Could you check a few things on this model? Use its own coordinates, in mm. A direction names the side the tool comes from. Coordinates: 2 decimals unless noted, no trailing zeros. Order: outer loops, then holes, each group sorted by start corner. A loop starts at its lowest first (then second) coordinate and runs counter-clockwise, first axis right, second up. Notation, with made-up numbers: (53.25, 62) -> (87.25, 62) arc R20 cw to (87.25, 86) -> close; hole circle Ø10 at (-29.5, 63.25). An arc over 180 degrees is marked (long way). Use a Markdown table: item, result. Add a question column.
1) Will these pins go through, and if not, where does the flat tip stop? pin 1 Ø1 at (x, z) = (1086.5, 212.5) entering from -Y; pin 2 Ø10 at (x, y) = (818, 769.5) entering from +Z; pin 3 Ø10 at (x, y) = (903.5, 157) entering from -Z; pin 4 Ø3 at (y, z) = (604, 85) entering from -X.
2) If I drill on L1, parallel to X at y = 150, z = 58.5; L2, parallel to Y at x = 3.5, z = 29; L3, parallel to X at y = 205.5, z = 50, over which ranges is the centre line in solid material (lowest first)? Write a range as [from, to].
3) If we section it at D-D (y = -7.5): Write out the boundary of the cut face in (x, z).
4) If we section it at B-B (z = 433): Write out the boundary of the cut face in (x, y), plus the area to 3 significant figures.
5) If we section it at C-C (x = 110.5): Write out the boundary of the cut face in (y, z), plus the area to 3 significant figures.
6) Which directions (+Z, -Z, +X, -X, +Y, -Y) give clear straight access to the entire face, cutting with the end or side of a thin tool? Please do faces 1 (the flat face through (-5, 607.5, 126)), 2 (the flat face through (1130, 759, 259)), 3 (the flat face through (1184, 439, 250)), 4 (the flat face through (305, 426.5, 139)).
7) If we section it at A-A (x = 883.5): Write out the boundary of the cut face in (y, z), plus the area to 3 significant figures.
8) Thinking about a two-plate mould opening in X: for faces 5 (the flat face through (794, 603, 139)), 6 (the flat face through (-25, 9, 251)), 7 (the flat face through (599, -25, 79)), which applies, +X half, -X half, draft (parallel to the pull), parting line (faces both ways), or undercut?
```python
from build123d import *

# Parameters (mm, degrees)
F0_W     = 179
F0_H     = 12
F0_W_2   = 138
F0_H_2   = 40
F0_W_3   = 40
F0_H_3   = 120
F0_W_4   = 92
F0_W_5   = 12
F0_H_4   = 90
F0_H_5   = 180
F0_W_6   = 87
F0_H_6   = 92
F0_W_7   = 26
F0_H_7   = 142
F0_H_8   = 136
F0_W_8   = 228
F0_H_9   = 18
F0_H_10  = 20
F0_W_9   = 20
F1_DEPTH = 5
F2_DEPTH = 277
F3_W     = 40
F3_H     = 120
F3_H_2   = 180
F4_DEPTH = 27
F6_DEPTH = 70
F7_DEPTH = 1265
F8_DEPTH = 70


with BuildPart() as f1:
    # F0 (on Top) → F1 (new body)
    with BuildSketch(Plane.XY):
        with Locations((1040.5, 269)):
            Rectangle(F0_W, F0_H)
        Polygon((794, 408), (794, 420), (669, 420), (669, 515), (652, 515), (652, 503), (657, 503), (657, 408), align=None)
        with Locations((392, -5)):
            Rectangle(F0_W_2, F0_H_2)
        Polygon((1130, 350), (1130, 530), (1130, 780), (806, 780), (806, 691), (832, 691), (832, 549), (806, 549), (806, 385), (806, 293), (806, 275), (839, 275), (859, 275), (951, 275), (1130, 275), align=None)
        with Locations((-5, 547.5)):
            Rectangle(F0_W_3, F0_H_3)
        with Locations((-5, 247.5)):
            Rectangle(F0_W_3, F0_H_3)
        Polygon((15, 487.5), (-25, 487.5), (-25, 307.5), (15, 307.5), (15, 382.1609020233), (15, 391.5), (15, 403.5), align=None)
        Polygon((15, 187.5), (-25, 187.5), (-25, -25), (323, -25), (323, 15), (15, 15), align=None)
        Polygon((1130, 15), (1130, 263), (951, 263), (859, 263), (839, 263), (839, 243), (839, 151), (839, 15), align=None)
        with Locations((905, 269)):
            Rectangle(F0_W_4, F0_H)
        Polygon((364.8940163038, 391.5), (243, 391.5), (243, 382.5), (364.8667633533, 382.5), align=None)
        Polygon((473, 780), (461, 780), (461, 498.5), (473, 498.5), (473, 503), (473, 515), align=None)
        with Locations((467, 453.5)):
            Rectangle(F0_W_5, F0_H_4)
        Polygon((243, 426.5), (243, 403.5), (364.9303535711, 403.5), (365, 426.5), align=None)
        Polygon((473, 503), (473, 498.5), (473, 408.5), (473, 386.5), (473, 296.5), (473, 275), (653, 275), (670, 275), (794, 275), (794, 293), (794, 385), (794, 408), (657, 408), (657, 503), (652, 503), (560, 503), align=None)
        with Locations((1150, 440)):
            Rectangle(F0_W_3, F0_H_5)
        Polygon((665, 263), (665, 15), (827, 15), (827, 151), (827, 243), (827, 263), (806, 263), (794, 263), align=None)
        with Locations((516.5, 509)):
            Rectangle(F0_W_6, F0_H)
        with Locations((467, 341.5)):
            Rectangle(F0_W_5, F0_H_4)
        Polygon((15, 382.1609020233), (15, 307.5), (15, 187.5), (15, 15), (323, 15), (461, 15), (461, 198.5), (435, 198.5), (435, 262.5), (461, 262.5), (461, 296.5), (461, 386.5), (461, 391.5), (365, 391.5), (364.8940163038, 391.5), (364.8667633533, 382.5), (243, 382.5), (243, 391.5), (15, 391.5), align=None)
        Polygon((1170, 530), (1170, 820), (-25, 820), (-25, 607.5), (15, 607.5), (15, 780), (461, 780), (473, 780), (794, 780), (806, 780), (1130, 780), (1130, 530), align=None)
        with Locations((833, 197)):
            Rectangle(F0_W_5, F0_H_6)
        Polygon((461, 198.5), (461, 15), (473, 15), (473, 275), (473, 296.5), (461, 296.5), (461, 262.5), (435, 262.5), (435, 198.5), align=None)
        Polygon((794, 420), (794, 780), (473, 780), (473, 515), (560, 515), (652, 515), (669, 515), (669, 420), align=None)
        with Locations((819, 620)):
            Rectangle(F0_W_7, F0_H_7)
        with Locations((606, 509)):
            Rectangle(F0_W_4, F0_H)
        with Locations((833, 83)):
            Rectangle(F0_W_5, F0_H_8)
        Polygon((653, 275), (653, 15), (665, 15), (665, 263), (794, 263), (794, 275), (670, 275), align=None)
        Polygon((1170, -25), (1170, 350), (1130, 350), (1130, 275), (1130, 263), (1130, 15), (839, 15), (827, 15), (665, 15), (653, 15), (473, 15), (461, 15), (461, -25), align=None)
        with Locations((800, 339)):
            Rectangle(F0_W_5, F0_H_6)
        with Locations((129, 397.5)):
            Rectangle(F0_W_8, F0_H)
        with Locations((800, 284)):
            Rectangle(F0_W_5, F0_H_9)
        Polygon((806, 691), (806, 780), (794, 780), (794, 420), (794, 408), (794, 385), (806, 385), (806, 549), align=None)
        with Locations((833, 253)):
            Rectangle(F0_W_5, F0_H_10)
        Polygon((839, 263), (839, 275), (806, 275), (806, 263), (827, 263), align=None)
        with Locations((849, 269)):
            Rectangle(F0_W_9, F0_H)
        Polygon((365, 403.5), (364.9303535711, 403.5), (364.8940163038, 391.5), (365, 391.5), (461, 391.5), (461, 386.5), (473, 386.5), (473, 408.5), (461, 408.5), (461, 403.5), align=None)
        Polygon((364.9303535711, 403.5), (243, 403.5), (243, 391.5), (364.8940163038, 391.5), align=None)
        with Locations((800, 269)):
            Rectangle(F0_W_5, F0_H)
        Polygon((15, 780), (15, 607.5), (15, 487.5), (15, 403.5), (243, 403.5), (243, 426.5), (365, 426.5), (364.9303535711, 403.5), (365, 403.5), (461, 403.5), (461, 408.5), (461, 498.5), (461, 780), align=None)
    extrude(amount=F1_DEPTH)

    # F0 (on Top) → F2 (join)
    with BuildSketch(Plane.XY):
        Polygon((15, 187.5), (-25, 187.5), (-25, -25), (323, -25), (323, 15), (15, 15), align=None)
        with Locations((392, -5)):
            Rectangle(F0_W_2, F0_H_2)
        Polygon((1170, -25), (1170, 350), (1130, 350), (1130, 275), (1130, 263), (1130, 15), (839, 15), (827, 15), (665, 15), (653, 15), (473, 15), (461, 15), (461, -25), align=None)
        with Locations((833, 83)):
            Rectangle(F0_W_5, F0_H_8)
        Polygon((653, 275), (653, 15), (665, 15), (665, 263), (794, 263), (794, 275), (670, 275), align=None)
        Polygon((461, 198.5), (461, 15), (473, 15), (473, 275), (473, 296.5), (461, 296.5), (461, 262.5), (435, 262.5), (435, 198.5), align=None)
        Polygon((15, 487.5), (-25, 487.5), (-25, 307.5), (15, 307.5), (15, 382.1609020233), (15, 391.5), (15, 403.5), align=None)
        with Locations((129, 397.5)):
            Rectangle(F0_W_8, F0_H)
        Polygon((243, 426.5), (243, 403.5), (364.9303535711, 403.5), (365, 426.5), align=None)
        Polygon((364.9303535711, 403.5), (243, 403.5), (243, 391.5), (364.8940163038, 391.5), align=None)
        Polygon((364.8940163038, 391.5), (243, 391.5), (243, 382.5), (364.8667633533, 382.5), align=None)
        Polygon((365, 403.5), (364.9303535711, 403.5), (364.8940163038, 391.5), (365, 391.5), (461, 391.5), (461, 386.5), (473, 386.5), (473, 408.5), (461, 408.5), (461, 403.5), align=None)
        Polygon((473, 780), (461, 780), (461, 498.5), (473, 498.5), (473, 503), (473, 515), align=None)
        with Locations((516.5, 509)):
            Rectangle(F0_W_6, F0_H)
        Polygon((794, 408), (794, 420), (669, 420), (669, 515), (652, 515), (652, 503), (657, 503), (657, 408), align=None)
        Polygon((806, 691), (806, 780), (794, 780), (794, 420), (794, 408), (794, 385), (806, 385), (806, 549), align=None)
        with Locations((833, 253)):
            Rectangle(F0_W_5, F0_H_10)
        with Locations((849, 269)):
            Rectangle(F0_W_9, F0_H)
        Polygon((839, 263), (839, 275), (806, 275), (806, 263), (827, 263), align=None)
        with Locations((800, 269)):
            Rectangle(F0_W_5, F0_H)
        with Locations((800, 284)):
            Rectangle(F0_W_5, F0_H_9)
        with Locations((1040.5, 269)):
            Rectangle(F0_W, F0_H)
        Polygon((1170, 530), (1170, 820), (-25, 820), (-25, 607.5), (15, 607.5), (15, 780), (461, 780), (473, 780), (794, 780), (806, 780), (1130, 780), (1130, 530), align=None)
        with Locations((819, 620)):
            Rectangle(F0_W_7, F0_H_7)
    extrude(amount=F2_DEPTH)

    # F3 (on face) → F4 (join)
    with BuildSketch(Plane.XY.offset(277)):
        with Locations((-5, 547.5)):
            Rectangle(F3_W, F3_H)
        with Locations((-5, 397.5)):
            Rectangle(F3_W, F3_H_2)
        with Locations((-5, 247.5)):
            Rectangle(F3_W, F3_H)
        with Locations((1150, 440)):
            Rectangle(F3_W, F3_H_2)
    extrude(amount=-F4_DEPTH)

    # F5 (on face) → F6 (join)
    with BuildSketch(Plane(origin=(-25, 0, 0), x_dir=(0, -1, 0), z_dir=(-1, 0, 0))):
        Polygon((-365.5990801838, 496), (-397.5, 496), (-125.3602941176, 277), (-93.4593743014, 277), align=None)
        Polygon((-93.4593743014, 277), (-125.3602941176, 277), (25, 156), (25, 181.6717461243), align=None)
        Polygon((25, 181.6717461243), (25, 156), (146.7794117647, 58), (159.3182351687, 73.5813320241), align=None)
        Polygon((-429.4009198162, 496), (-397.5, 496), (-365.5990801838, 496), (-397.5, 521.6717461243), align=None)
        Polygon((-669.6397058824, 277), (-397.5, 496), (-429.4009198162, 496), (-701.5406256986, 277), align=None)
        Polygon((-941.7794117647, 58), (-820, 156), (-820, 181.6717461243), (-954.3182351687, 73.5813320241), align=None)
        Polygon((-820, 156), (-669.6397058824, 277), (-701.5406256986, 277), (-820, 181.6717461243), align=None)
    extrude(amount=F6_DEPTH)

    # F7 (add, through all): a face of the model
    f7_faces = [f1.faces().sort_by_distance(p)[0] for p in [
        (-95, 117.7974560425, 286.3979384905),
    ]]
    extrude(f7_faces, amount=-F7_DEPTH)

    # F8 (add): a face of the model
    f8_faces = [f1.faces().sort_by_distance(p)[0] for p in [
        (1170, 807.7023270544, 229.3358730621),
    ]]
    extrude(f8_faces, amount=F8_DEPTH)


solid = f1.part
```
Answer sheet:
| question | item | result |
|---|---|---|
| 1 | pin 1 | y = -25 |
| 1 | pin 2 | z = 226.33 |
| 1 | pin 3 | z = 0 |
| 1 | pin 4 | x = 461 |
| 2 | L1 | [-25, 15], [461, 473], [653, 665], [827, 839], [1130, 1240] |
| 2 | L2 | [-25, 187.5], [307.5, 487.5], [607.5, 820] |
| 2 | L3 | [435, 473], [653, 665], [1130, 1240] |
| 3 | outline | (-95, 170.08) -> (-25, 170.08) -> (-25, 0) -> (1240, 0) -> (1240, 277) -> (-25, 277) -> (-25, 195.75) -> (-95, 195.75) -> close |
| 4 | outline | (-95, 287.31) -> (1240, 287.31) -> (1240, 319.21) -> (-95, 319.21) -> close; (-95, 475.79) -> (1240, 475.79) -> (1240, 507.69) -> (-95, 507.69) -> close |
| 4 | area | 85,200 mm2 |
| 5 | outline | (-159.32, 73.58) -> (-146.78, 58) -> (-25, 156) -> (-25, 0) -> (820, 0) -> (820, 156) -> (941.78, 58) -> (954.32, 73.58) -> (820, 181.67) -> (820, 277) -> (780, 277) -> (780, 213.86) -> (397.5, 521.67) -> (15, 213.86) -> (15, 277) -> (-25, 277) -> (-25, 181.67) -> close; hole (15, 5) -> (391.5, 5) -> (391.5, 277) -> (403.5, 277) -> (403.5, 5) -> (780, 5) -> (780, 188.19) -> (397.5, 496) -> (15, 188.19) -> close |
| 5 | area | 55,500 mm2 |
| 6 | face 1 | -X |
| 6 | face 2 | +Z |
| 6 | face 3 | +X |
| 6 | face 4 | none |
| 7 | outline | (-159.32, 73.58) -> (-146.78, 58) -> (-25, 156) -> (-25, 0) -> (820, 0) -> (820, 156) -> (941.78, 58) -> (954.32, 73.58) -> (820, 181.67) -> (820, 277) -> (780, 277) -> (780, 213.86) -> (397.5, 521.67) -> (15, 213.86) -> (15, 277) -> (-25, 277) -> (-25, 181.67) -> close; hole (15, 5) -> (780, 5) -> (780, 188.19) -> (397.5, 496) -> (15, 188.19) -> close |
| 7 | area | 52,200 mm2 |
| 8 | face 5 | undercut |
| 8 | face 6 | -X half |
| 8 | face 7 | draft |
